Work out the finished part from the listing and answer in its coordinate system (mm). A direction names the side the tool comes from. Give positions to 0.01 mm unless a question says otherwise; leave off trailing zeros. Loops run counter-clockwise (first coordinate to the right, second up) from the corner with the lowest first, then second, coordinate; pieces in that order, holes last.
```python
from build123d import *

# Parameters (mm, degrees)
SKETCH_1_W          = 75
SKETCH_1_H          = 60
EXTRUDE_1_DEPTH     = 4
SKETCH_2_W          = 3.2
SKETCH_2_H          = 15
CUT_EXTRUDE_1_DEPTH = 97.13012015
CUT_EXTRUDE_2_DEPTH = 97.13012015
CHAMFER_1_SIZE      = 15
SKETCH_7_W          = 10
SKETCH_7_H          = 30
EXTRUDE_3_DEPTH     = 4
SKETCH_8_W          = 3.2
SKETCH_8_H          = 15
CUT_EXTRUDE_5_DEPTH = 105.120122935
FILLET_1_R          = 5
EXTRUDE_2_DEPTH     = 3


with BuildPart() as part:
    # 草图1 → 凸台-拉伸1 (new body)
    with BuildSketch(Plane.XY):
        with Locations((37.5, 30)):
            Rectangle(SKETCH_1_W, SKETCH_1_H)
    extrude(amount=EXTRUDE_1_DEPTH)

    # 草图2 → 切除-拉伸1 (cut, through all)
    with BuildSketch(Plane.XY.offset(4)):
        with Locations((66, 30)):
            Rectangle(SKETCH_2_W, SKETCH_2_H)
        with Locations((9, 30)):
            Rectangle(SKETCH_2_W, SKETCH_2_H)
    extrude(amount=-CUT_EXTRUDE_1_DEPTH, mode=Mode.SUBTRACT)

    # 草图3 → 切除-拉伸2 (cut, through all)
    with BuildSketch(Plane.XY.offset(4)):
        with BuildLine():
            Line((58.9, 48.5), (58.9, 44.5))
            Line((58.9, 44.5), (61.4, 44.5))
            Line((61.4, 44.5), (61.4, 48.5))
            ThreePointArc((61.4, 48.5), (60.15, 51.098749218), (58.9, 48.5))
        make_face()
        with BuildLine():
            Line((58.9, 15.5), (61.4, 15.5))
            Line((61.4, 15.5), (61.4, 11.5))
            ThreePointArc((61.4, 11.5), (60.15, 8.901250782), (58.9, 11.5))
            Line((58.9, 11.5), (58.9, 15.5))
        make_face()
        with BuildLine():
            Line((16.1, 15.5), (16.1, 11.5))
            ThreePointArc((16.1, 11.5), (14.85, 8.901250782), (13.6, 11.5))
            Line((13.6, 11.5), (13.6, 15.5))
            Line((13.6, 15.5), (16.1, 15.5))
        make_face()
        with BuildLine():
            Line((13.6, 48.5), (13.6, 44.5))
            Line((13.6, 44.5), (16.1, 44.5))
            Line((16.1, 44.5), (16.1, 48.5))
            ThreePointArc((16.1, 48.5), (14.85, 51.098749218), (13.6, 48.5))
        make_face()
    extrude(amount=-CUT_EXTRUDE_2_DEPTH, mode=Mode.SUBTRACT)

    # 倒角1
    chamfer_1_edges = [part.edges().sort_by_distance(p)[0] for p in [
        (0, 60, 2),
        (75, 60, 2),
        (75, 0, 2),
        (0, 0, 2),
    ]]
    chamfer(chamfer_1_edges, length=CHAMFER_1_SIZE)

    # 草图7 → 凸台-拉伸3 (add)
    with BuildSketch(Plane.XY.offset(4)):
        with Locations((-5, 30)):
            Rectangle(SKETCH_7_W, SKETCH_7_H)
        with Locations((80, 30)):
            Rectangle(SKETCH_7_W, SKETCH_7_H)
    extrude(amount=-EXTRUDE_3_DEPTH)

    # 草图8 → 切除-拉伸5 (cut, through all)
    with BuildSketch(Plane.XY.offset(4)):
        with Locations((79.75, 30)):
            Rectangle(SKETCH_8_W, SKETCH_8_H)
        with Locations((-4.75, 30)):
            Rectangle(SKETCH_8_W, SKETCH_8_H)
    extrude(amount=-CUT_EXTRUDE_5_DEPTH, mode=Mode.SUBTRACT)

    # 圆角1
    fillet_1_edges = [part.edges().sort_by_distance(p)[0] for p in [
        (0, 15, 2),
        (0, 45, 2),
        (60, 60, 2),
        (15, 60, 2),
        (75, 45, 2),
        (75, 15, 2),
        (15, 0, 2),
        (60, 0, 2),
        (-10, 45, 2),
        (-10, 15, 2),
        (85, 15, 2),
        (85, 45, 2),
    ]]
    fillet(fillet_1_edges, radius=FILLET_1_R)

    # 草图5 → 凸台-拉伸2 (add)
    with BuildSketch(Plane(origin=(0, 0, 0), x_dir=(-1, 0, 0), z_dir=(0, 0, -1))):
        Polygon((-37.5, 42.5), (-79.4, 42.5), (-79.4, 38.5), (-39.5, 38.5), (-39.5, 21.5), (-79.4, 21.5), (-79.4, 17.5), (-37.5, 17.5), align=None)
        Polygon((4.4, 42.5), (-37.5, 42.5), (-37.5, 17.5), (4.4, 17.5), (4.4, 21.5), (-35.5, 21.5), (-35.5, 38.5), (4.4, 38.5), align=None)
    extrude(amount=EXTRUDE_2_DEPTH)


solid = part.part
```
Q1. Given pin 1 (0.9 mm diameter, centred on y = 30.5, z = -1.5, fed in from -X); pin 2 (0.9 mm diameter, centred on x = 50, z = -1, fed in from +Y); pin 3 (2 mm diameter, centred on y = 10.5, z = -0.5, fed in from +X), each flat-ended and moving along its own axis, determine where each tip first touches the part or whether it passes through.
Q2. Section C-C on y = 36.5 is taken. Give the vertices of the cut face in (x, z), plus the area to 3 significant figures.
Q3. Section B-B on x = 34.5 is taken. Give the vertices of the cut face in (y, z).
Q4. Section A-A on y = 47.5 is taken. Give the vertices of the cut face in (x, z).
Q5. Consider line 1 along X through (y, z) = (30, 3.5); line 2 along Y through (x, z) = (28, -1.5); line 3 along X through (y, z) = (49, 1). Determine where each line is inside the solid, lowest interval first.
Q6. Section D-D on z = -1.25 is taken. Give the vertices of the cut face in (x, y), plus the area to 3 significant figures.
Q7. Which of the six approach directions +Z, -Z, +X, -X, +Y, -Y give full straight-line access (tool end or side, diameter ignored) to faces 1 (the face through (79, 45, 2)), 2 (the face through (60, 44.5, 2)), 3 (the face through (79.4, 41, -1))?
Q8. Determine the mould class of faces 4 (the face through (13.6, 47, 2)), 5 (the face through (79.4, 20, -1)), 6 (the face through (-4, 45, 2)) for opening direction Y: +Y half, -Y half, draft (parallel to the pull), parting line (faces both ways), or undercut.
Check result:
1. pin 1: stops at x = 35.5
1. pin 2: stops at y = 42.5
1. pin 3: stops at x = 71.37
2. outline: (-10, 0) - (-6.35, 0) - (-6.35, 4) - (-10, 4) - close; (-3.15, 0) - (7.4, 0) - (7.4, 4) - (-3.15, 4) - close; (10.6, 0) - (35.5, 0) - (35.5, -3) - (39.5, -3) - (39.5, 0) - (64.4, 0) - (64.4, 4) - (10.6, 4) - close; (67.6, 0) - (78.15, 0) - (78.15, 4) - (67.6, 4) - close; (81.35, 0) - (85, 0) - (85, 4) - (81.35, 4) - close
2. area: 341 mm2
3. outline: (0, 0) - (17.5, 0) - (17.5, -3) - (21.5, -3) - (21.5, 0) - (38.5, 0) - (38.5, -3) - (42.5, -3) - (42.5, 0) - (60, 0) - (60, 4) - (0, 4) - close
4. outline: (2.5, 0) - (13.6, 0) - (13.6, 4) - (2.5, 4) - close; (16.1, 0) - (58.9, 0) - (58.9, 4) - (16.1, 4) - close; (61.4, 0) - (72.5, 0) - (72.5, 4) - (61.4, 4) - close
5. line 1: x = -10 to -6.35, -3.15 to 7.4, 10.6 to 64.4, 67.6 to 78.15, 81.35 to 85
5. line 2: y = 17.5 to 21.5, 38.5 to 42.5
5. line 3: x = 4 to 13.33, 16.37 to 58.63, 61.67 to 71
6. outline: (-4.4, 17.5) - (79.4, 17.5) - (79.4, 21.5) - (39.5, 21.5) - (39.5, 38.5) - (79.4, 38.5) - (79.4, 42.5) - (-4.4, 42.5) - (-4.4, 38.5) - (35.5, 38.5) - (35.5, 21.5) - (-4.4, 21.5) - close
6. area: 738 mm2
7. face 1: +Z, -Z, +X, +Y
7. face 2: +Z, -Z
7. face 3: -Z, +X, +Y, -Y
8. face 4: undercut
8. face 5: draft
8. face 6: +Y half
